```python
from build123d import *

# Parameters (mm, degrees)
F0_W     = 3.000019
F0_H     = 10.000005
F0_W_2   = 2.999994
F1_DEPTH = 3.048


with BuildPart() as f1:
    # F0 (on Front) → F1 (new body)
    with BuildSketch(Plane.XZ):
        Polygon((-74.500003, 64.499998), (-74.500003, 14.999995), (-80.499991, 14.999995), (-80.499991, -10.000005), (-74.500003, -10.000005), (-74.500003, -64.500023), (-64.999997, -64.500023), (-64.999997, -67.500017), (-54.999992, -67.500017), (-54.999992, -64.500023), (-34.999981, -64.500023), (-34.999981, -67.500017), (-25.000001, -67.500017), (-25.000001, -64.500023), (-4.99999, -64.500023), (-4.99999, -67.500017), (5.000015, -67.500017), (5.000015, -64.500023), (25.000001, -64.500023), (25.000001, -67.500017), (35.000006, -67.500017), (35.000006, -64.500023), (55.000017, -64.500023), (55.000017, -67.500017), (64.999997, -67.500017), (64.999997, -64.500023), (74.500003, -64.500023), (74.500003, -10.000005), (80.500017, -10.000005), (80.500017, 14.999995), (74.500003, 14.999995), (74.500003, 64.499998), (55.000017, 64.499998), (55.000017, 67.499992), (45.000012, 67.499992), (45.000012, 64.499998), (5.000015, 64.499998), (5.000015, 67.499992), (-4.99999, 67.499992), (-4.99999, 64.499998), (-44.999986, 64.499998), (-44.999986, 67.499992), (-54.999992, 67.499992), (-54.999992, 64.499998), align=None)
        with Locations((-72.999993, 2.499982)):
            Rectangle(F0_W, F0_H, mode=Mode.SUBTRACT)
        with Locations((73.000006, 2.499982)):
            Rectangle(F0_W_2, F0_H, mode=Mode.SUBTRACT)
    extrude(amount=F1_DEPTH)


solid = f1.part
```
The model under review builds one solid part; all positions refer to its coordinate system, in mm. Round coordinates to 2 decimals unless told otherwise and drop trailing zeros. Loops run counter-clockwise (first coordinate to the right, second up) from the corner with the lowest first, then second, coordinate; pieces in that order, holes last.
Item 1: For line 1 (X direction, y = -1.1, z = 4); line 2 (Z direction, x = 72.5, y = -2.4); line 3 (Z direction, x = -56.5, y = -1.55), list the stretches that pass through material, from the lowest coordinate up.
Determined:
line 1: x = -80.5 to -74.5, -71.5 to 71.5, 74.5 to 80.5
line 2: z = -64.5 to -2.5, 7.5 to 64.5
line 3: z = -67.5 to 64.5
Item 2: Clearance check with flat-ended pins moving along their axes: pin 1 Ø0.9 at (y, z) = (-1.5, -65.5) entering from +X; pin 2 Ø1.5 at (y, z) = (-1.5, 66.5) entering from -X; pin 3 Ø1.5 at (x, y) = (-71.5, -2) entering from -Z; pin 4 Ø3 at (x, z) = (14.5, 15.5) entering from +Y. State where each tip first meets the part, or that it passes through.
Determined:
pin 1: stops at x = 65
pin 2: stops at x = -55
pin 3: stops at z = -64.5
pin 4: stops at y = 0
Item 3: Take a section at A-A (x = 12). Write out the cut boundary in (y, z), then the cut area to 3 significant figures.
Determined:
outline: (-3.05, -64.5) - (0, -64.5) - (0, 64.5) - (-3.05, 64.5) - close
area: 393 mm2
Item 4: Take a section at B-B (y = -0.6). Give the number of separate pieces and of enclosed holes in the cut face, then the cut area to 3 significant figures.
Determined:
separate pieces: 1
enclosed holes: 2
area: 19,700 mm2
Item 5: Take a section at C-C (z = -22). Write out the cut boundary in (x, y).
Determined:
outline: (-74.5, -3.05) - (74.5, -3.05) - (74.5, 0) - (-74.5, 0) - close
